Geometry: see drawing. Coordinates: mm, zero at the bounding-box minimum. Round coordinates to 2 decimals unless told otherwise and drop trailing zeros. Order: outer loops, then holes, each group sorted by start corner. A loop starts at its lowest first (then second) coordinate and runs counter-clockwise, first axis right, second up. Notation, with made-up numbers: M 87,3.25 L 140,3.25 A7 ccw 140,8.25 Z; hole C 0,29 d1. An arc over 180 degrees is marked long. Answer in a Markdown table with one row per item. Add a question column.
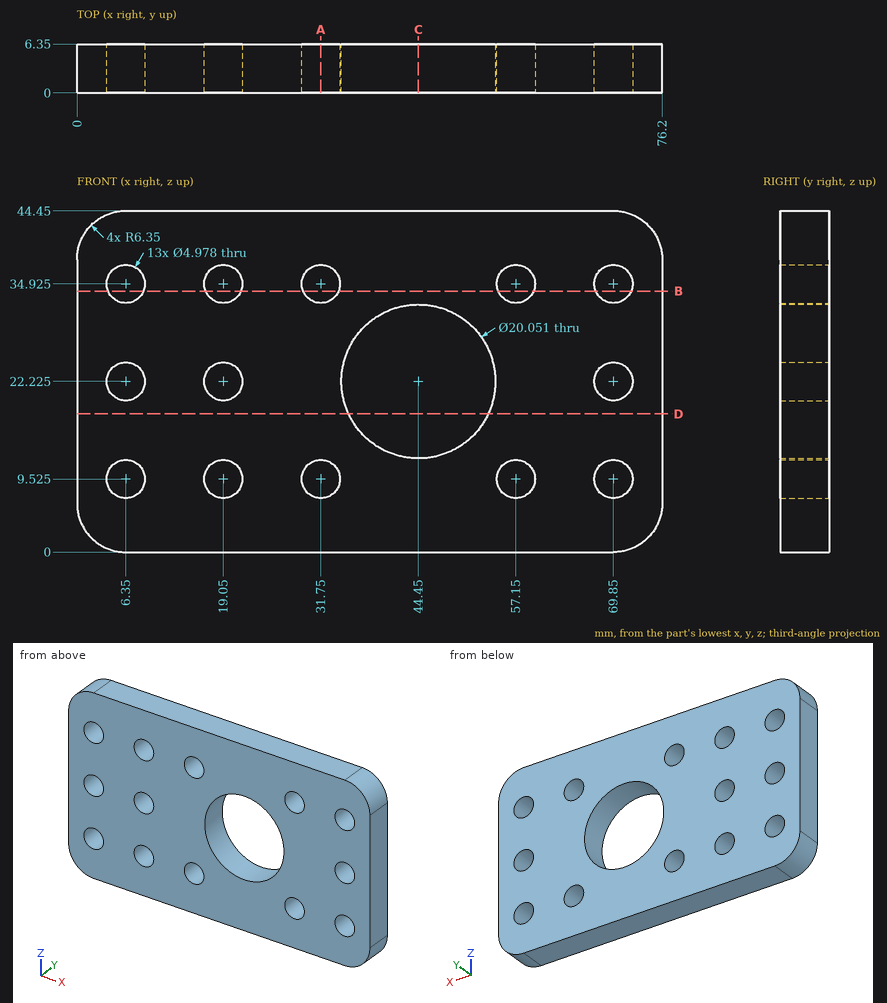
(1) Line query: line 1 (Z direction, x = 6.5, y = 2.5); line 2 (X direction, y = 0.5, z = 22.5); line 3 (Z direction, x = 44.5, y = 3.5). Output: solid intervals per line, ascending. Write a range as from..to.
(2) Cut plane A-A (x = 31.75). Count the separate pieces of the cut face and the enclosed holes in it, and give its area (3 significant figures).
(3) Pin query (flat end, axial travel): pin 1 (4.5 mm diameter, centred on x = 6.35, z = 34.925, fed in from -Y) (1 decimal); pin 2 (2 mm diameter, centred on y = 3.5, z = 39.5, fed in from -X). Return the tip coordinate at first contact, or that it passes through.
(4) Cut plane B-B (z = 34). Return loops of the section in (x, y), and give its area (3 significant figures).
(5) Cut plane C-C (x = 44.45). Return loops of the section in (y, z), and give its area (3 significant figures).
(6) Cut plane D-D (z = 18). Return loops of the section in (x, y).
Answer list:
| question | item | result |
|---|---|---|
| 1 | line 1 | 0..7.04, 12.01..19.74, 24.71..32.44, 37.41..44.45 |
| 1 | line 2 | 0..3.88, 8.82..16.58, 21.52..34.43, 54.47..67.38, 72.32..76.2 |
| 1 | line 3 | 0..12.2, 32.25..44.45 |
| 2 | separate pieces | 3 |
| 2 | enclosed holes | 0 |
| 2 | area | 219 mm² |
| 3 | pin 1 | through |
| 3 | pin 2 | x = 0.01 |
| 4 | outline | M 0,0 L 4.04,0 L 4.04,6.35 L 0,6.35 Z; M 8.66,0 L 16.74,0 L 16.74,6.35 L 8.66,6.35 Z; M 21.36,0 L 29.44,0 L 29.44,6.35 L 21.36,6.35 Z; M 34.06,0 L 54.84,0 L 54.84,6.35 L 34.06,6.35 Z; M 59.46,0 L 67.54,0 L 67.54,6.35 L 59.46,6.35 Z; M 72.16,0 L 76.2,0 L 76.2,6.35 L 72.16,6.35 Z |
| 4 | area | 337 mm² |
| 5 | outline | M 0,0 L 6.35,0 L 6.35,12.2 L 0,12.2 Z; M 0,32.25 L 6.35,32.25 L 6.35,44.45 L 0,44.45 Z |
| 5 | area | 155 mm² |
| 6 | outline | M 0,0 L 35.36,0 L 35.36,6.35 L 0,6.35 Z; M 53.54,0 L 76.2,0 L 76.2,6.35 L 53.54,6.35 Z |
